Geometry: see drawing. Coordinates: mm, zero at the bounding-box minimum. A direction names the side the tool comes from. Coordinates: 2 decimals unless noted, no trailing zeros. Order: outer loops, then holes, each group sorted by start corner. A loop starts at its lowest first (then second) coordinate and runs counter-clockwise, first axis right, second up. Notation, with made-up numbers: (-10.75, 32) -> (21.25, 32) arc R20 ccw to (21.25, 67) -> close; hole circle Ø7 at (66, -1.5). An arc over 180 degrees is marked (long way). Write each question's results on one line, items separated by ' | '. Start each with the question number.
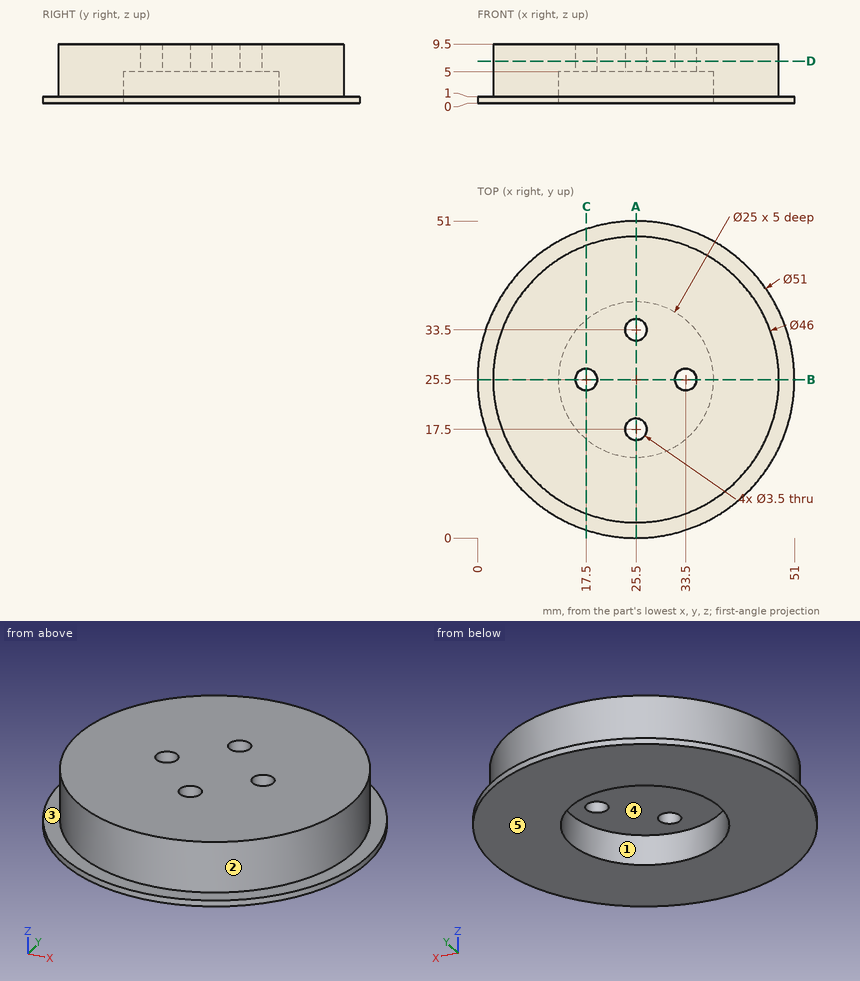
(1) Line query: L1, parallel to Y at x = 25.5, z = 7.8; L2, parallel to X at y = 24.5, z = 7.25; L3, parallel to Y at x = 27.5, z = 2.5. Output: solid intervals per line, ascending.
(2) First-contact query: P1, Ø1.5, axis at y = 41, z = 2, coming from the +X side; P2, Ø7.5, axis at x = 24, y = 31.5, coming from the -Z side; P3, Ø3, axis at x = 17.5, y = 25.5, coming from the -Z side; P4, Ø2, axis at x = 31, z = 8.5, coming from the +Y side. Flat tips, straight axial feed; report the tip coordinate or a pass-through.
(3) Section D-D on z = 6.75. Return the cut outline in (x, y).
(4) Reachability of the marked faces 4 and 5 from +Z, -Z, +X, -X, +Y, -Y: full face, straight path, thin tool, end or side. Return the list, or none.
(5) Section C-C on x = 17.5. Return the cut outline in (y, z), then the cut area to 3 significant figures.
(6) Section A-A on x = 25.5. Return the cut outline in (y, z).
(7) Draft query along Y for the marked faces 1, 2 and 3. Return one class per face: released by +Y, released by -Y, zero draft, split by the parting line, or undercut.
Results list:
1) L1: y = 2.5 to 15.75, 19.25 to 31.75, 35.25 to 48.5 | L2: x = 2.52 to 16.06, 18.94 to 32.06, 34.94 to 48.48 | L3: y = 2.59 to 13.16, 37.84 to 48.41
2) P1: stops at x = 43.15 | P2: stops at z = 5 | P3: passes through | P4: stops at y = 48.06
3) outline: circle Ø46 at (25.5, 25.5); hole circle Ø3.5 at (17.5, 25.5); hole circle Ø3.5 at (25.5, 17.5); hole circle Ø3.5 at (25.5, 33.5); hole circle Ø3.5 at (33.5, 25.5)
4) face 4: -Z | face 5: -Z, +X, -X, +Y, -Y
5) outline: (1.29, 0) -> (15.9, 0) -> (15.9, 5) -> (23.75, 5) -> (23.75, 9.5) -> (3.94, 9.5) -> (3.94, 1) -> (1.29, 1) -> close; (27.25, 5) -> (35.1, 5) -> (35.1, 0) -> (49.71, 0) -> (49.71, 1) -> (47.06, 1) -> (47.06, 9.5) -> (27.25, 9.5) -> close | area: 303 mm²
6) outline: (0, 0) -> (13, 0) -> (13, 5) -> (15.75, 5) -> (15.75, 9.5) -> (2.5, 9.5) -> (2.5, 1) -> (0, 1) -> close; (19.25, 5) -> (31.75, 5) -> (31.75, 9.5) -> (19.25, 9.5) -> close; (35.25, 5) -> (38, 5) -> (38, 0) -> (51, 0) -> (51, 1) -> (48.5, 1) -> (48.5, 9.5) -> (35.25, 9.5) -> close
7) face 1: undercut | face 2: split by the parting line | face 3: zero draft
